Model file for the job. Use its own axes, mm. A direction names the side the tool comes from. Round coordinates to 2 decimals unless told otherwise and drop trailing zeros. Loops run counter-clockwise (first coordinate to the right, second up) from the corner with the lowest first, then second, coordinate; pieces in that order, holes last. Notation, with made-up numbers: (55.25, 29) - (82.25, 29) arc R33 ccw to (82.25, 68) - close; hole circle Ø5 at (5, 50). An arc over 180 degrees is marked (long way). Answer as a JSON object with one key per item and string values.
from build123d import *

# Parameters (mm, degrees)
BOSS_EXTRUDE1_DEPTH         = 4.7625
F_3_4_0_75_DIAMETER_HOLE1_D = 19.05
SKETCH4_W                   = 11.1125
SKETCH4_H                   = 18.415
CUT_EXTRUDE1_DEPTH          = 5.7625
F_6_CLEARANCE_HOLE1_D       = 4.3053


with BuildPart() as part:
    # Sketch1 → Boss-Extrude1 (new body)
    with BuildSketch(Plane.XY):
        Polygon((-44.1325, -84.1375), (-30.7975, -108.1405), (-1.5875, -108.1405), (-1.5875, 26.9875), (-44.1325, 26.9875), align=None)
    extrude(amount=BOSS_EXTRUDE1_DEPTH)

    # 3/4 (0.75) Diameter Hole1 (through all)
    with Locations(Plane.XY.offset(4.7625)):
        with Locations((-31.4325, -1.620345612), (-17.4625, -86.5505), (-22.86, -53.5305)):
            Hole(F_3_4_0_75_DIAMETER_HOLE1_D / 2)

    # Sketch4 → Cut-Extrude1 (cut, through all)
    with BuildSketch(Plane.XY.offset(4.7625)):
        with Locations((-12.7, -6.0325)):
            Rectangle(SKETCH4_W, SKETCH4_H)
    extrude(amount=-CUT_EXTRUDE1_DEPTH, mode=Mode.SUBTRACT)

    # #6 Clearance Hole1 (through all)
    with Locations(Plane.XY.offset(4.7625)):
        with Locations((-36.3855, -80.4545), (-12.7, 19.05), (-31.4325, 21.404754388), (-31.4325, -24.620045612)):
            Hole(F_6_CLEARANCE_HOLE1_D / 2)


solid = part.part
1) Probe probe 1 along Y at (x, z) = (-23.5, 1.7); probe 2 along Y at (x, z) = (-13, 2.35) (1 decimal); probe 3 along Y at (x, z) = (-21, 1.55). List the from-to ranges inside material, lowest first.
Values follow:
{"probe 1": "-108.14 to -93.92, -79.18 to -63.03, -44.03 to -6.89, 3.65 to 26.99", "probe 2": "-108.1 to -95, -78.1 to -15.2, 3.2 to 16.9, 21.2 to 27", "probe 3": "-108.14 to -95.39, -77.71 to -62.87, -44.19 to 26.99"}
2) Drop flat-ended pins along their axis: P1, Ø3.5, axis at x = -12.7, y = 19.05, coming from the +Z side; P2, Ø2, axis at y = -87.5, z = 2, coming from the -X side. Give the stop position or say it passes through.
Values follow:
{"P1": "through", "P2": "x = -42.82"}
3) Slice it at A-A on x = -25.5. List the corners of the cut face in (y, z).
Values follow:
{"outline": "(-108.14, 0) - (-91.66, 0) - (-91.66, 4.76) - (-108.14, 4.76) - close; (-81.44, 0) - (-62.68, 0) - (-62.68, 4.76) - (-81.44, 4.76) - close; (-44.38, 0) - (-9.07, 0) - (-9.07, 4.76) - (-44.38, 4.76) - close; (5.83, 0) - (26.99, 0) - (26.99, 4.76) - (5.83, 4.76) - close"}
4) Slice it at B-B on z = 1.5. Count the separate pieces of the cut face and the enclosed holes in it, then the cut area to 3 significant figures.
Values follow:
{"separate pieces": "1", "enclosed holes": "8", "area": "4,470 mm²"}
5) Two-plate mould, pull along Y, no slides. Class faces 3 (the cylindrical face through (-34.235, -80.36, 2.348)), 4 (the flat face through (-7.144, -6, 2)), 5 (the flat face through (-1.588, -42, 2)), 6 (the flat face through (-37.56, -95.97, 2.35)): pulls with the +Y half, pulls with the -Y half, needs draft (parallel to the pull), parting line crosses it, or undercut.
Values follow:
{"face 3": "undercut", "face 4": "undercut", "face 5": "needs draft", "face 6": "pulls with the -Y half"}
6) Tool access for faces 1 (the flat face through (-13, -15.24, 2)), 2 (the flat face through (-23, 26.988, 2)): list every direction of +Z, -Z, +X, -X, +Y, -Y with a clear straight run to the whole face (end or side of a thin tool).
Values follow:
{"face 1": "+Z, -Z", "face 2": "+Z, -Z, +X, -X, +Y"}
